Can you work these out from the model? Positions are in its coordinate system, mm. A direction names the side the tool comes from. Round coordinates to 2 decimals unless told otherwise and drop trailing zeros. Order: outer loops, then holes, each group sorted by start corner. A loop starts at its lowest first (then second) coordinate and runs counter-clockwise, first axis right, second up.
Autodesk Inventor part; units mm, degrees
ref_plane "YZ Plane" through (0, 0, 0) normal (1, 0, 0) x (0, 1, 0)
ref_plane "XZ Plane" through (0, 0, 0) normal (0, 1, 0) x (-1, 0, 0)
ref_plane "XY Plane" through (0, 0, 0) normal (0, 0, 1) x (1, 0, 0)
ref_plane "Work Plane1" through (0, -11.6382, 33.3368) normal (0, 0, 1) x (1, 0, 0)
sketch "Sketch7" plane through (0, -11.6382, 33.3368) normal (0, 0, 1) x (1, 0, 0)
  line L0 (0, 15.5588) -> (27, 15.5588)
  line L1 (27, 15.5588) -> (27, 17.5588)
  line L2 (27, 17.5588) -> (0, 27.386)
  line L3 (0, 27.386) -> (0, 15.5588)
  line L4 (0, 15.5588) -> (27, 15.5588)
  point P0 (0, 11.6382)
  dimension "d20" = 2
  dimension "d21" = 110
  dimension "d76" = 27
extrude "Extrusion5" add sketch "Sketch7" against normal blind 67
sketch "Sketch8" plane through (0, 3.9206, 33.3368) normal (-1, 0, 0) x (0, 0, 1)
  line L0 (0, 0) -> (-67, 0)
  line L1 (-67, 0) -> (0, -24.386)
  line L2 (0, -24.386) -> (0, 0)
  point P0 (-33.3368, -3.9206)
  dimension "d27" = 20
extrude "Extrusion6" add sketch "Sketch8" against normal up to surface (27 mm away)
shell "Shell3" thickness 3 removed faces 1 at (9, -4.2081, -11.3299)
sketch "Sketch9" plane through (27, 5.9206, 33.3368) normal (0.3420201, 0.9396926, 0) x (0.9396926, -0.3420201, 0)
  line L0 (-21.711, 26.8228) -> (-7.711, 26.8228)
  line L1 (-7.711, 26.8228) -> (-7.711, 40.8228)
  line L2 (-7.711, 40.8228) -> (-21.711, 40.8228)
  line L3 (-21.711, 40.8228) -> (-21.711, 26.8228)
  line L4 (-7.711, 33.8228) -> (47.289, 33.8228) construction
  line L5 (-15.1557, 3.6455) -> (-2, 8.4338)
  line L6 (-2, 8.4338) -> (-6.7883, 21.5895)
  line L7 (-6.7883, 21.5895) -> (-19.944, 16.8012)
  line L8 (-19.944, 16.8012) -> (-15.1557, 3.6455)
  line L9 (-19.944, 50.8443) -> (-6.7883, 46.056)
  line L10 (-6.7883, 46.056) -> (-2, 59.2117)
  line L11 (-2, 59.2117) -> (-15.1557, 64)
  line L12 (-15.1557, 64) -> (-19.944, 50.8443)
  line L13 (0, 0) -> (0, 67)
  line L14 (-28.7328, 67) -> (0, 67)
  point P0 (-4.3941, 15.0117)
  point P1 (-4.3941, 52.6339)
  dimension "d31" = 14
  dimension "d32" = 55
  dimension "d35" = 20
  dimension "d39" = 20
  dimension "d41" = 2
  dimension "d42" = 3
extrude "Extrusion7" cut sketch "Sketch9" against normal up to next
fillet "Fillet1" radius 4 1 edges at (0, 15.7478, -0.1632)
sketch "Sketch10" plane through (27, 5.9206, 33.3368) normal (1, 0, 0) x (0, 0, -1)
  line L0 (0, -26.386) -> (67, -2)
  line L1 (41.6283, -11.2345) -> (40.6022, -8.4155)
  line L2 (40.6022, -8.4155) -> (51.8786, -4.3112)
  line L3 (51.8786, -4.3112) -> (52.9046, -7.1303)
  point P0 (33.3368, -5.9206)
  dimension "d46" = 3
  dimension "d47" = 12
  dimension "d48" = 15
ref_plane "Work Plane2" through (13.5, 5.9206, 33.3368) normal (1, 0, 0) x (0, 0, -1)
extrude "Extrusion8" add sketch "Sketch10" along normal blind 6
sketch "Sketch11" plane through (27, -2.4949, -7.2655) normal (0, 0.9396926, 0.3420201) x (1, 0, 0)
  line L0 (0, 0) -> (6, 0)
  line L1 (6, 12) -> (6, 0)
  point P0 (-27, -5.974)
  point P1 (3, 5)
  dimension "d52" = 5
  dimension "d53" = 3
hole "Hole1" at (30, -0.7848, -11.9639) direction (0, -0.9396926, -0.3420201) diameter 3 end through all
mirror "Mirror2" about plane through (13.5, 5.9206, 33.3368) normal (1, 0, 0) of "Extrusion8", "Hole1"
sketch "Sketch12" plane through (0, 3.9206, -33.6632) normal (0, -0.9396926, -0.3420201) x (1, 0, 0)
  line L0 (3, 68.1074) -> (24, 68.1074)
  line L1 (10.5, 68.1074) -> (16.5, 68.1074)
  line L2 (16.5, 68.1074) -> (16.5, 75.063)
  line L3 (16.5, 75.063) -> (10.5, 75.063)
  line L4 (10.5, 75.063) -> (10.5, 68.1074)
  line L5 (27, 0) -> (0, 0)
  line L6 (27, 71.2999) -> (27, 27)
  point P0 (0, 32.974)
  dimension "d61" = 75.063
  dimension "d62" = 6
  dimension "d64" = 10.5
extrude "Extrusion9" add sketch "Sketch12" against normal blind 3
sketch "Sketch13" plane through (0, 6.7397, -32.6372) normal (0, 0.9396926, 0.3420201) x (1, 0, 0)
  line L0 (10.5, -75.063) -> (16.5, -75.063)
  line L1 (16.5, -75.063) -> (16.5, -70.208)
  point P0 (0, -32.974)
  point P1 (13.5, -72.063)
  dimension "d67" = 3
  dimension "d68" = 3
hole "Hole2" at (13.5, -17.9073, 35.0799) direction (0, -0.9396926, -0.3420201) diameter 3 end through all
properties part number "k2_t_l1a"
(1) On a 3-axis mill with a long thin cutter (end or side, diameter ignored), from which of +Z, -Z, +X, -X, +Y, -Y can I reach the whole of each face in a straight line? I mean faces 4 (the face through (29.958, 0.22, -19.048)), 5 (the face through (3, 0, 7)), 6 (the face through (-2.958, 0.042, -14.235)), 7 (the face through (-6, -2, -14)), 8 (the face through (-2.087, -1.807, -13.603)). Say none if no direction works.
(2) I want a section at D-D, the plane x = 1. List the corners of the cut face in (y, z) for me, plus the area to 3 significant figures.
(3) If we mould it in two halves opening along Z, with no side actions, what happens to faces 1 (the face through (29.958, -3.924, -7.786)), 2 (the face through (6.092, 11.956, -0.584)), 3 (the face through (10, 8, -33.663))? For each: pulls with the +Z half, pulls with the -Z half, needs draft (parallel to the pull), parting line crosses it, or undercut.
(4) I want a section at C-C, the plane z = 21. List the corners of the cut face in (x, y) for me.
(5) Please list where these lines run through material, in increasing order: probe 1 along X at (y, z) = (1, -9); probe 2 along Z at (x, y) = (3.5, 2); probe 3 along X at (y, z) = (-16, 30.5).
(6) I want a section at A-A, the plane z = 4.5. List the corners of the cut face in (x, y) for me.
(7) I want a section at B-B, the plane y = -13.5. List the corners of the cut face in (x, z) for me.
(8) I'm going to push flat-ended pins straight in: pin 1 Ø2 at (y, z) = (-18.5, 35.5) entering from -X; pin 2 Ø12 at (y, z) = (9, 10) entering from +X; pin 3 Ø4 at (x, y) = (13, 8) entering from +Z; pin 4 Ø21 at (y, z) = (-6, -0.5) entering from +X. Where does each tip first touch, or does it pass through?
Ans:
1. face 4: -Z, +X, +Y
1. face 5: -Y
1. face 6: +Z, -X, +Y
1. face 7: +Z, -Z, -X, +Y, -Y
1. face 8: none
2. outline: (-20.47, 33.34) - (3.92, -33.66) - (12.68, -33.66) - (12.68, 33.34) - close
2. area: 1,400 mm2
3. face 1: pulls with the +Z half
3. face 2: undercut
3. face 3: pulls with the -Z half
4. outline: (0, -15.98) - (3, -15.98) - (3, 11.46) - (8.76, 9.37) - (9.79, 12.19) - (5.37, 13.79) arc R4 ccw to (0, 10.04) - close; (22.76, 4.27) - (24, 3.82) - (24, -15.98) - (27, -15.98) - (27, 5.92) - (23.79, 7.09) - close
5. probe 1: x = 0 to 3, 24 to 27
5. probe 2: z = 30.34 to 33.34
5. probe 3: x = 0 to 27
6. outline: (0, -9.97) - (3, -9.97) - (3, 11.46) - (5.57, 10.53) - (6.6, 13.35) - (5.37, 13.79) arc R4 ccw to (0, 10.04) - close; (18.73, 5.74) - (24, 3.82) - (24, -9.97) - (27, -9.97) - (27, 5.92) - (19.75, 8.56) - close
7. outline: (0, 14.2) - (3, 14.2) - (3, 30.34) - (24, 30.34) - (24, 14.2) - (27, 14.2) - (27, 33.34) - (0, 33.34) - close
8. pin 1: stops at x = 10.5
8. pin 2: stops at x = 27
8. pin 3: stops at z = 33.34
8. pin 4: stops at x = 33
